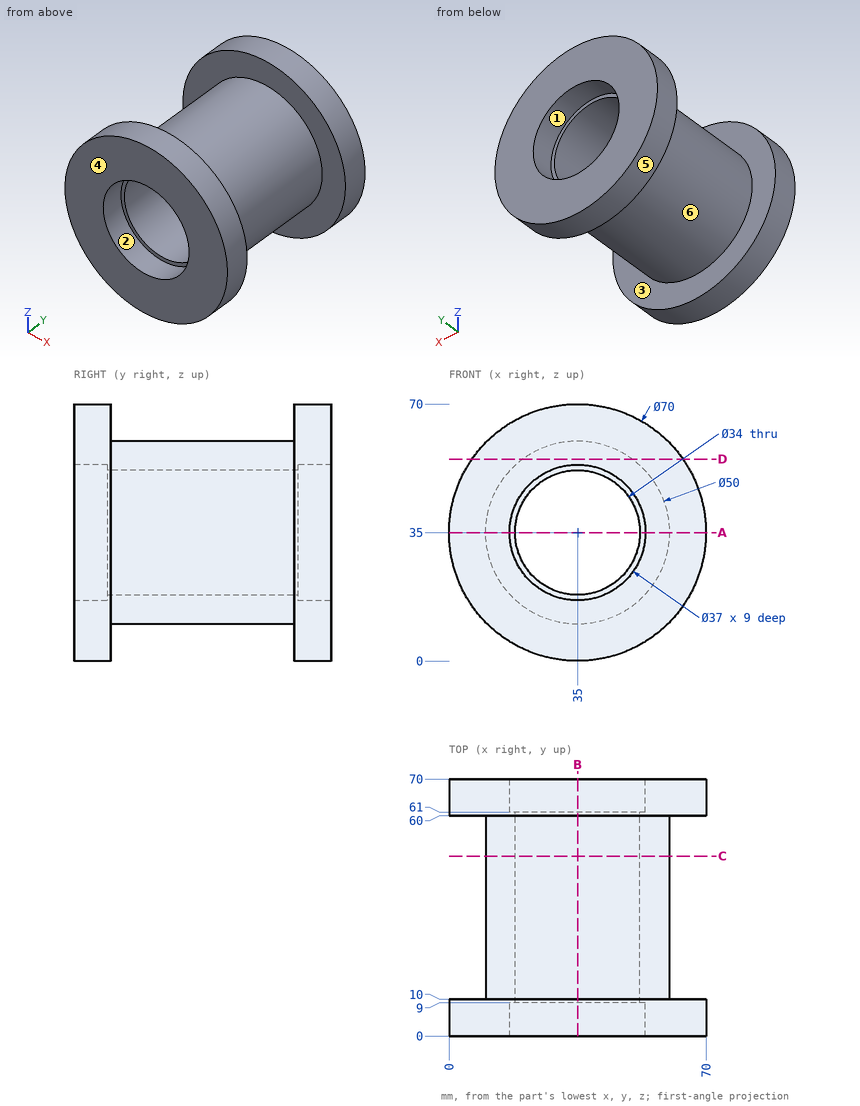
Could you check a few things on this drawing? It's one solid part, dimensions in mm from its lowest x, y, z. A direction names the side the tool comes from. Give positions to 0.01 mm unless a question says otherwise; leave off trailing zeros. Order: outer loops, then holes, each group sorted by start corner. A loop starts at its lowest first (then second) coordinate and runs counter-clockwise, first axis right, second up. Notation, with made-up numbers: (13.25, -33.5) -> (37.25, -33.5) arc R21 ccw to (37.25, -12.5) -> close; hole circle Ø11 at (19.25, 75.5). An arc over 180 degrees is marked (long way). Use CSV: the item, a comma, the result in double quotes. Start each with the question number.
Item 1: Suppose I cut it at A-A (z = 35). List the corners of the cut face in (x, y) for me.
Item 2: Suppose I cut it at C-C (y = 49). List the corners of the cut face in (x, z) for me.
Item 3: Suppose I cut it at D-D (z = 55). List the corners of the cut face in (x, y) for me.
Item 4: Thinking about a two-plate mould opening in Y: for the marked faces 4, 5 and 6, which applies, pulls with the +Y half, pulls with the -Y half, needs draft (parallel to the pull), parting line crosses it, or undercut?
Item 5: Suppose I cut it at B-B (x = 35). List the corners of the cut face in (y, z) for me.
Item 6: I'm going to push flat-ended pins straight in: P1, Ø1.5, axis at x = 17, y = 38.5, coming from the +Z side; P2, Ø6, axis at y = 44, z = 14.5, coming from the +X side; P3, Ø10, axis at x = 19, y = 27, coming from the +Z side; P4, Ø1.5, axis at x = 8.5, z = 20, coming from the -Y side. Where does each tip first touch, or does it pass through?
Item 7: If I drill on probe 1 along X at (y, z) = (64, 35); probe 2 along Y at (x, z) = (60, 38); probe 3 along Z at (x, y) = (33, 20), over which ranges is the centre line in solid material (lowest first)? Write a range as [from, to].
Item 8: On a 3-axis mill with a long thin cutter (end or side, diameter ignored), from which of +Z, -Z, +X, -X, +Y, -Y can I reach the whole of each face in a straight line? I mean the marked faces 1, 2 and 3. Say none if no direction works.
Answer block:
1,outline,"(0, 0) -> (16.5, 0) -> (16.5, 9) -> (18, 9) -> (18, 61) -> (16.5, 61) -> (16.5, 70) -> (0, 70) -> (0, 60) -> (10, 60) -> (10, 10) -> (0, 10) -> close; (52, 9) -> (53.5, 9) -> (53.5, 0) -> (70, 0) -> (70, 10) -> (60, 10) -> (60, 60) -> (70, 60) -> (70, 70) -> (53.5, 70) -> (53.5, 61) -> (52, 61) -> close"
2,outline,"circle Ø50 at (35, 35); hole circle Ø34 at (35, 35)"
3,outline,"(6.28, 0) -> (63.72, 0) -> (63.72, 10) -> (50, 10) -> (50, 60) -> (63.72, 60) -> (63.72, 70) -> (6.28, 70) -> (6.28, 60) -> (20, 60) -> (20, 10) -> (6.28, 10) -> close"
4,face 4,"pulls with the -Y half"
4,face 5,"needs draft"
4,face 6,"undercut"
5,outline,"(0, 0) -> (10, 0) -> (10, 10) -> (60, 10) -> (60, 0) -> (70, 0) -> (70, 16.5) -> (61, 16.5) -> (61, 18) -> (9, 18) -> (9, 16.5) -> (0, 16.5) -> close; (0, 53.5) -> (9, 53.5) -> (9, 52) -> (61, 52) -> (61, 53.5) -> (70, 53.5) -> (70, 70) -> (60, 70) -> (60, 60) -> (10, 60) -> (10, 70) -> (0, 70) -> close"
6,P1,"stops at z = 53.1"
6,P2,"stops at x = 52.85"
6,P3,"stops at z = 57.45"
6,P4,"stops at y = 0"
7,probe 1,"x = [0, 16.5], [53.5, 70]"
7,probe 2,"y = [0, 10], [60, 70]"
7,probe 3,"z = [10.08, 18.12], [51.88, 59.92]"
8,face 1,"+Y"
8,face 2,"-Y"
8,face 3,"none"
